Check sheet for the modelled part. Datum: model origin and axes. Units: mm. A direction names the side the tool comes from. Give positions to 0.01 mm unless a question says otherwise; leave off trailing zeros. Order: outer loops, then holes, each group sorted by start corner. A loop starts at its lowest first (then second) coordinate and runs counter-clockwise, first axis right, second up.
from build123d import *

# Parameters (mm, degrees)
SKETCH001_W   = 34
SKETCH001_H   = 38
SKETCH001_R   = 1.5
SKETCH001_W_2 = 12.3
SKETCH001_H_2 = 23.1
EXTRUDE_DEPTH = 1.5
FILLET_R      = 1


with BuildPart() as part:
    # Sketch001 → Extrude (new body)
    with BuildSketch(Plane.XY):
        Rectangle(SKETCH001_W, SKETCH001_H)
        with Locations((0, 14.1)):
            Circle(SKETCH001_R, mode=Mode.SUBTRACT)
        with Locations((0, -14.1)):
            Circle(SKETCH001_R, mode=Mode.SUBTRACT)
        with Locations((13.5, 15.5)):
            Circle(SKETCH001_R, mode=Mode.SUBTRACT)
        with Locations((-13.5, 15.5)):
            Circle(SKETCH001_R, mode=Mode.SUBTRACT)
        with Locations((-13.5, -15.5)):
            Circle(SKETCH001_R, mode=Mode.SUBTRACT)
        with Locations((13.5, -15.5)):
            Circle(SKETCH001_R, mode=Mode.SUBTRACT)
        Rectangle(SKETCH001_W_2, SKETCH001_H_2, mode=Mode.SUBTRACT)
    extrude(amount=EXTRUDE_DEPTH)

    # Fillet
    fillet_edges = [part.edges().sort_by_distance(p)[0] for p in [
        (-17, 19, 0.75),
        (17, 19, 0.75),
        (17, -19, 0.75),
        (-17, -19, 0.75),
    ]]
    fillet(fillet_edges, radius=FILLET_R)


solid = part.part
1) Depth check by flat-ended pin: pin 1 Ø3.5 at (x, y) = (0, 14.1) entering from +Z; pin 2 Ø10 at (x, y) = (1, -4) entering from -Z. Enter the tip coordinate at first touch or a pass-through.
Recorded:
pin 1: stops at z = 1.5
pin 2: passes through
2) Set-up check for faces 4 (the face through (-16.715, 18.699, 0.76)), 5 (the face through (0, -11.55, 1)): record each of +Z, -Z, +X, -X, +Y, -Y from which the full face is reachable in a straight line by a thin tool's end or side.
Recorded:
face 4: +Z, -Z, -X, +Y
face 5: +Z, -Z
3) Section check A-A, the plane y = 2.5. Record the cut outline in (x, z), then the cut area to 4 significant figures.
Recorded:
outline: (-17, 0) - (-6.15, 0) - (-6.15, 1.5) - (-17, 1.5) - close; (6.15, 0) - (17, 0) - (17, 1.5) - (6.15, 1.5) - close
area: 32.55 mm2
4) Material ranges on L1, parallel to Y at x = 13.5, z = 0.45; L2, parallel to Y at x = 0, z = 0.55; L3, parallel to Y at x = -12.5, z = 0.7, recorded low to high.
Recorded:
L1: y = -19 to -17, -14 to 14, 17 to 19
L2: y = -19 to -15.6, -12.6 to -11.55, 11.55 to 12.6, 15.6 to 19
L3: y = -19 to -16.62, -14.38 to 14.38, 16.62 to 19
5) Draft check along Y on faces 1 (the face through (0, 19, 1)), 2 (the face through (12, 15.57, 0.74)), 3 (the face through (17, 0, 1)). Enter one of: +Y half, -Y half, draft (parallel to the pull), parting line (faces both ways), or undercut.
Recorded:
face 1: +Y half
face 2: undercut
face 3: draft
6) Section check D-D, the plane x = 13.5. Record the cut outline in (y, z).
Recorded:
outline: (-19, 0) - (-17, 0) - (-17, 1.5) - (-19, 1.5) - close; (-14, 0) - (14, 0) - (14, 1.5) - (-14, 1.5) - close; (17, 0) - (19, 0) - (19, 1.5) - (17, 1.5) - close
7) Section check C-C, the plane z = 1. Record the cut outline in (x, y).
Recorded:
outline: (-17, -18) arc R1 ccw to (-16, -19) - (16, -19) arc R1 ccw to (17, -18) - (17, 18) arc R1 ccw to (16, 19) - (-16, 19) arc R1 ccw to (-17, 18) - close; hole circle Ø3 at (-13.5, -15.5); hole circle Ø3 at (-13.5, 15.5); hole (-6.15, -11.55) - (6.15, -11.55) - (6.15, 11.55) - (-6.15, 11.55) - close; hole circle Ø3 at (0, -14.1); hole circle Ø3 at (0, 14.1); hole circle Ø3 at (13.5, -15.5); hole circle Ø3 at (13.5, 15.5)
8) Section check B-B, the plane x = -5. Record the cut outline in (y, z).
Recorded:
outline: (-19, 0) - (-11.55, 0) - (-11.55, 1.5) - (-19, 1.5) - close; (11.55, 0) - (19, 0) - (19, 1.5) - (11.55, 1.5) - close
